from build123d import *

# Parameters (mm, degrees)
SKETCH_1_R          = 20
EXTRUDE_1_DEPTH     = 3
CUT_EXTRUDE_1_REACH = 30.443
SKETCH_2_R          = 1.15
CUT_EXTRUDE_2_REACH = 30.443
SKETCH_3_R          = 1.65
SKETCH_3_R_2        = 5


with BuildPart() as part:
    # 草图1 → 凸台-拉伸1 (new body)
    with BuildSketch(Plane(origin=(0, 0, 0), x_dir=(1, 0, 0), z_dir=(0, 1, 0))):
        with Locations(Location((0, 0, 0), (0, 0, 270))):
            Circle(SKETCH_1_R)
    extrude(amount=EXTRUDE_1_DEPTH)

    # 草图2 → 切除-拉伸1 (cut, up to next)
    with BuildSketch(Plane(origin=(0, 3, 0), x_dir=(1, 0, 0), z_dir=(0, 1, 0)), mode=Mode.PRIVATE) as cut_extrude_1_sk1:
        with Locations(Location((0, 16.75, 0), (0, 0, 270))):
            Circle(SKETCH_2_R)
    cut_extrude_1_tool1 = extrude(cut_extrude_1_sk1.sketch, amount=-CUT_EXTRUDE_1_REACH, mode=Mode.PRIVATE) & part.part
    # 草图2 → 切除-拉伸1 (cut, up to next)
    with BuildSketch(Plane(origin=(0, 3, 0), x_dir=(1, 0, 0), z_dir=(0, 1, 0)), mode=Mode.PRIVATE) as cut_extrude_1_sk2:
        with Locations(Location((16.75, 0, 0), (0, 0, 270))):
            Circle(SKETCH_2_R)
    cut_extrude_1_tool2 = extrude(cut_extrude_1_sk2.sketch, amount=-CUT_EXTRUDE_1_REACH, mode=Mode.PRIVATE) & part.part
    # 草图2 → 切除-拉伸1 (cut, up to next)
    with BuildSketch(Plane(origin=(0, 3, 0), x_dir=(1, 0, 0), z_dir=(0, 1, 0)), mode=Mode.PRIVATE) as cut_extrude_1_sk3:
        with Locations(Location((0, -16.75, 0), (0, 0, 270))):
            Circle(SKETCH_2_R)
    cut_extrude_1_tool3 = extrude(cut_extrude_1_sk3.sketch, amount=-CUT_EXTRUDE_1_REACH, mode=Mode.PRIVATE) & part.part
    # 草图2 → 切除-拉伸1 (cut, up to next)
    with BuildSketch(Plane(origin=(0, 3, 0), x_dir=(1, 0, 0), z_dir=(0, 1, 0)), mode=Mode.PRIVATE) as cut_extrude_1_sk4:
        with Locations(Location((-16.75, 0, 0), (0, 0, 270))):
            Circle(SKETCH_2_R)
    cut_extrude_1_tool4 = extrude(cut_extrude_1_sk4.sketch, amount=-CUT_EXTRUDE_1_REACH, mode=Mode.PRIVATE) & part.part
    add(cut_extrude_1_tool1.solids().sort_by_distance((0, 3, -16.75))[0], mode=Mode.SUBTRACT)
    add(cut_extrude_1_tool2.solids().sort_by_distance((16.75, 3, 0))[0], mode=Mode.SUBTRACT)
    add(cut_extrude_1_tool3.solids().sort_by_distance((0, 3, 16.75))[0], mode=Mode.SUBTRACT)
    add(cut_extrude_1_tool4.solids().sort_by_distance((-16.75, 3, 0))[0], mode=Mode.SUBTRACT)

    # 草图3 → 切除-拉伸2 (cut, up to next)
    with BuildSketch(Plane(origin=(0, 3, 0), x_dir=(1, 0, 0), z_dir=(0, 1, 0)), mode=Mode.PRIVATE) as cut_extrude_2_sk1:
        with Locations(Location((-9.5, 0, 0), (0, 0, 270))):
            Circle(SKETCH_3_R)
    cut_extrude_2_tool1 = extrude(cut_extrude_2_sk1.sketch, amount=-CUT_EXTRUDE_2_REACH, mode=Mode.PRIVATE) & part.part
    # 草图3 → 切除-拉伸2 (cut, up to next)
    with BuildSketch(Plane(origin=(0, 3, 0), x_dir=(1, 0, 0), z_dir=(0, 1, 0)), mode=Mode.PRIVATE) as cut_extrude_2_sk2:
        with Locations(Location((9.5, 0, 0), (0, 0, 270))):
            Circle(SKETCH_3_R)
    cut_extrude_2_tool2 = extrude(cut_extrude_2_sk2.sketch, amount=-CUT_EXTRUDE_2_REACH, mode=Mode.PRIVATE) & part.part
    # 草图3 → 切除-拉伸2 (cut, up to next)
    with BuildSketch(Plane(origin=(0, 3, 0), x_dir=(1, 0, 0), z_dir=(0, 1, 0)), mode=Mode.PRIVATE) as cut_extrude_2_sk3:
        with Locations(Location((0, 0, 0), (0, 0, 270))):
            Circle(SKETCH_3_R_2)
    cut_extrude_2_tool3 = extrude(cut_extrude_2_sk3.sketch, amount=-CUT_EXTRUDE_2_REACH, mode=Mode.PRIVATE) & part.part
    add(cut_extrude_2_tool1.solids().sort_by_distance((-9.5, 3, 0))[0], mode=Mode.SUBTRACT)
    add(cut_extrude_2_tool2.solids().sort_by_distance((9.5, 3, 0))[0], mode=Mode.SUBTRACT)
    add(cut_extrude_2_tool3.solids().sort_by_distance((0, 3, 0))[0], mode=Mode.SUBTRACT)


solid = part.part
Could you check a few things on this model? Use its own coordinates, in mm. Give positions to 0.01 mm unless a question says otherwise; leave off trailing zeros. Order: outer loops, then holes, each group sorted by start corner. A loop starts at its lowest first (then second) coordinate and runs counter-clockwise, first axis right, second up. Notation, with made-up numbers: (37.5, 10) -> (42.5, 10) arc R19 cw to (42.5, 21) -> close; hole circle Ø7 at (59, 2.5). An arc over 180 degrees is marked (long way). Answer in a Markdown table with one row per item. Add a question column.
Item 1: Imagine slicing it at B-B (y = 2.05). List the corners of the cut face in (x, z) for me.
Item 2: We'd pull the mould along Y, two halves only. Please class faces 1 (the cylindrical face through (-11.1, 1.5, -0.4)), 2 (the flat face through (-4, 0, 4)), 3 (the flat face through (-4, 3, 4)): pulls with the +Y half, pulls with the -Y half, needs draft (parallel to the pull), parting line crosses it, or undercut.
Item 3: I'm going to push flat-ended pins straight in: P1, Ø3.5, axis at x = 0, z = 16.75, coming from the -Y side; P2, Ø1, axis at x = 13.5, y = 1.5, coming from the +Z side. Where does each tip first touch, or does it pass through?
Item 4: Please list where these lines run through material, in increasing order: probe 1 along X at (y, z) = (1, 0); probe 2 along Z at (x, y) = (1, 2.4); probe 3 along Z at (x, y) = (9, 2.5).
Item 5: Imagine slicing it at C-C (z = -16.75). List the corners of the cut face in (x, y) for me, and give its area (3 significant figures).
Item 6: Imagine slicing it at D-D (x = 9.5). List the corners of the cut face in (y, z) for me.
Item 7: Imagine slicing it at A-A (x = 0). List the corners of the cut face in (y, z) for me.
Result:
| question | item | result |
|---|---|---|
| 1 | outline | circle Ø40 at (0, 0); hole circle Ø2.3 at (-16.75, 0); hole circle Ø3.3 at (-9.5, 0); hole circle Ø10 at (0, 0); hole circle Ø2.3 at (0, -16.75); hole circle Ø2.3 at (0, 16.75); hole circle Ø3.3 at (9.5, 0); hole circle Ø2.3 at (16.75, 0) |
| 2 | face 1 | needs draft |
| 2 | face 2 | pulls with the -Y half |
| 2 | face 3 | pulls with the +Y half |
| 3 | P1 | y = 0 |
| 3 | P2 | z = 15.2 |
| 4 | probe 1 | -20 to -17.9, -15.6 to -11.15, -7.85 to -5, 5 to 7.85, 11.15 to 15.6, 17.9 to 20 |
| 4 | probe 2 | -19.97 to -17.32, -16.18 to -4.9, 4.9 to 16.18, 17.32 to 19.97 |
| 4 | probe 3 | -17.86 to -1.57, 1.57 to 17.86 |
| 5 | outline | (-10.93, 0) -> (-1.15, 0) -> (-1.15, 3) -> (-10.93, 3) -> close; (1.15, 0) -> (10.93, 0) -> (10.93, 3) -> (1.15, 3) -> close |
| 5 | area | 58.7 mm2 |
| 6 | outline | (0, -17.6) -> (3, -17.6) -> (3, -1.65) -> (0, -1.65) -> close; (0, 1.65) -> (3, 1.65) -> (3, 17.6) -> (0, 17.6) -> close |
| 7 | outline | (0, -20) -> (3, -20) -> (3, -17.9) -> (0, -17.9) -> close; (0, -15.6) -> (3, -15.6) -> (3, -5) -> (0, -5) -> close; (0, 5) -> (3, 5) -> (3, 15.6) -> (0, 15.6) -> close; (0, 17.9) -> (3, 17.9) -> (3, 20) -> (0, 20) -> close |
